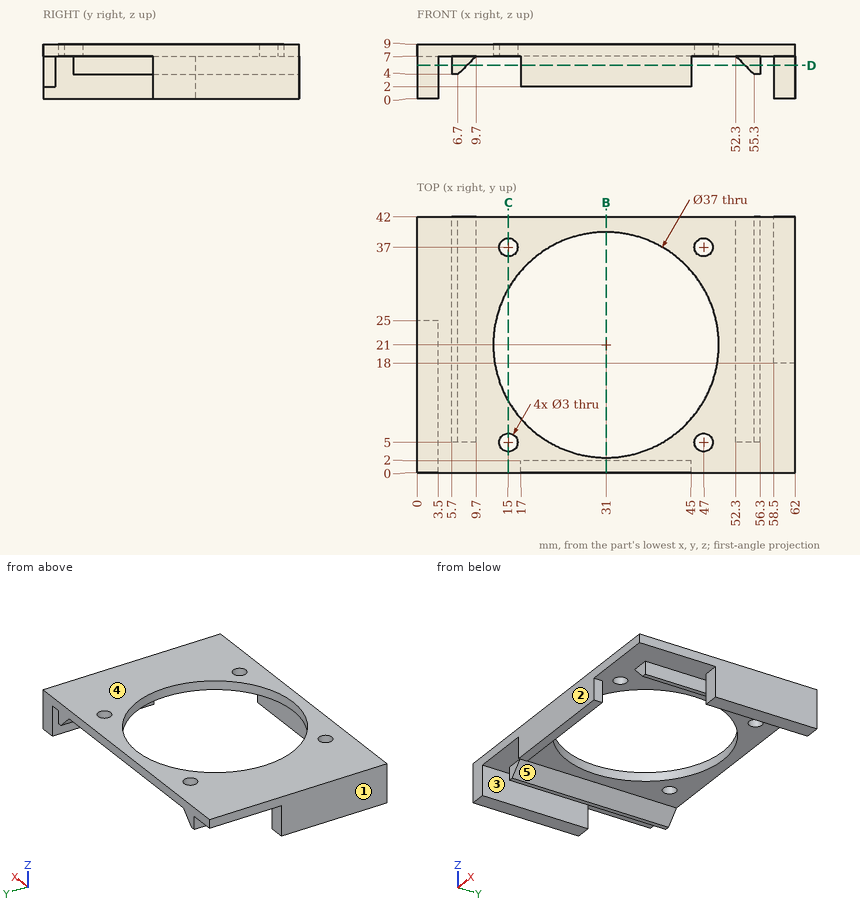
Geometry: see drawing. Coordinates: mm, zero at the bounding-box minimum. A direction names the side the tool comes from. Coordinates: 2 decimals unless noted, no trailing zeros. Loops run counter-clockwise (first coordinate to the right, second up) from the corner with the lowest first, then second, coordinate; pieces in that order, holes last.
(1) Pull-direction query (X, two-part tool) for the marked faces 1, 2 and 3; classes: released by +X, released by -X, zero draft, split by the parting line, or undercut.
(2) Section D-D on z = 5.5. Return the cut outline in (x, y).
(3) Material intervals for probe 1 along X at (y, z) = (19, 6); probe 2 along Y at (x, z) = (48, 7.5); probe 3 along Y at (x, z) = (47, 8.6), sorted ascending.
(4) First-contact query: pin 1 Ø3 at (x, z) = (1.5, 4.5) entering from +Y; pin 2 Ø2.5 at (x, y) = (15, 37) entering from +Z; pin 3 Ø0.9 at (x, z) = (7, 5.5) entering from -Y; pin 4 Ø0.8 at (x, y) = (56, 30) entering from -Z. Flat tips, straight axial feed; report the tip coordinate or a pass-through.
(5) Section C-C on x = 15. Return the cut outline in (y, z).
(6) Set-up query: the marked faces 4 and 5. Return all of +Z, -Z, +X, -X, +Y, -Y with unobstructed straight access to the full face (end or side cutting, diameter ignored); none if empty.
(7) Section B-B on x = 31. Return the cut outline in (y, z).
Data:
1. face 1: released by -X
1. face 2: zero draft
1. face 3: undercut
2. outline: (0, 0) - (3.5, 0) - (3.5, 25) - (0, 25) - close; (5.7, 5) - (8.2, 5) - (8.2, 42) - (5.7, 42) - close; (17, 0) - (45, 0) - (45, 2) - (17, 2) - close; (53.8, 5) - (56.3, 5) - (56.3, 42) - (53.8, 42) - close; (58.5, 18) - (62, 18) - (62, 42) - (58.5, 42) - close
3. probe 1: x = 0 to 3.5, 5.7 to 8.7, 53.3 to 56.3, 58.5 to 62
3. probe 2: y = 0 to 3.88, 6.12 to 13.7, 28.3 to 35.88, 38.12 to 42
3. probe 3: y = 0 to 3.5, 6.5 to 11.71, 30.29 to 35.5, 38.5 to 42
4. pin 1: stops at y = 25
4. pin 2: passes through
4. pin 3: stops at y = 5
4. pin 4: stops at z = 4
5. outline: (0, 7) - (3.5, 7) - (3.5, 9) - (0, 9) - close; (6.5, 7) - (11.71, 7) - (11.71, 9) - (6.5, 9) - close; (30.29, 7) - (35.5, 7) - (35.5, 9) - (30.29, 9) - close; (38.5, 7) - (42, 7) - (42, 9) - (38.5, 9) - close
6. face 4: +Z, +X, -X, +Y, -Y
6. face 5: -Z, +Y, -Y
7. outline: (0, 2) - (2, 2) - (2, 7) - (2.5, 7) - (2.5, 9) - (0, 9) - close; (39.5, 7) - (42, 7) - (42, 9) - (39.5, 9) - close
